Geometry: see drawing. Coordinates: mm, zero at the bounding-box minimum. Round coordinates to 2 decimals unless told otherwise and drop trailing zeros. Loops run counter-clockwise (first coordinate to the right, second up) from the corner with the lowest first, then second, coordinate; pieces in that order, holes last. Notation, with made-up numbers: M 75.5,2.5 L 109.5,2.5 A19 cw 109.5,13.5 Z; hole C -7.5,51 d8. An arc over 180 degrees is marked long. Answer as a JSON object with one key per item and string values.
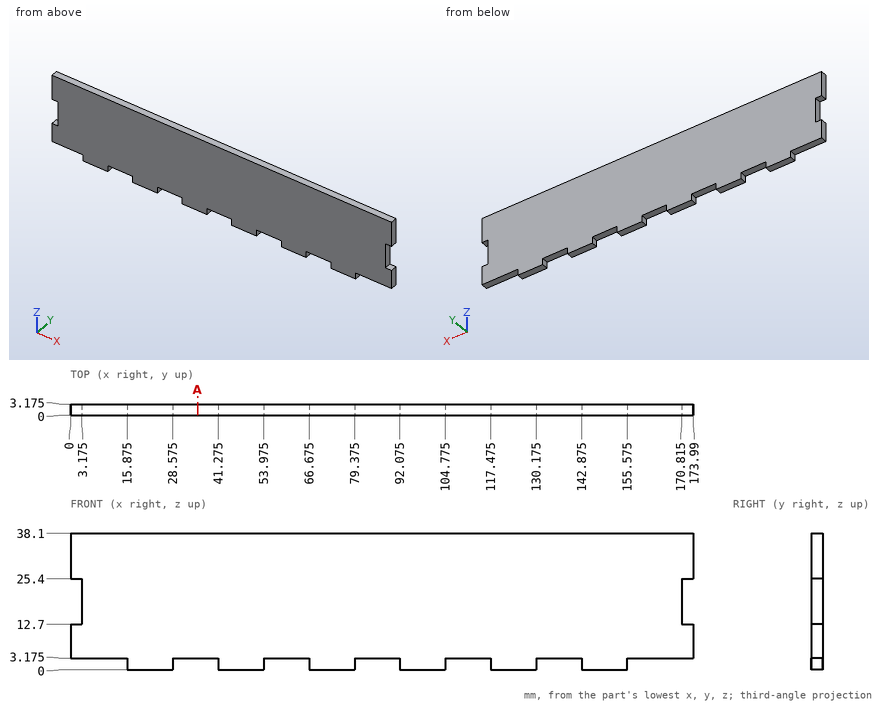
1) Pin query (flat end, axial travel): P1, Ø1, axis at y = 1, z = 1, coming from the -X side (3 decimals); P2, Ø1, axis at y = 0.5, z = 24.5, coming from the -X side (3 decimals); P3, Ø1.6, axis at y = 2, z = 2, coming from the +X side (3 decimals). Return the tip coordinate at first contact, or that it passes through.
Results:
{"P1": "x = 15.875", "P2": "x = 3.175", "P3": "x = 155.575"}
2) Ray query, line 1 (Z direction, x = 61.5, y = 0.5) (3 decimals); line 2 (X direction, y = 2.4, z = 21) (3 decimals). Return the intervals inside material, ascending.
Results:
{"line 1": "3.175 to 38.1", "line 2": "3.175 to 170.815"}
3) Section query A-A (x = 35.5). Return the cut outline in (y, z) (3 decimals).
Results:
{"outline": "M 0,3.175 L 3.175,3.175 L 3.175,38.1 L 0,38.1 Z"}
